```python
from build123d import *
from build123d.topology import SkipClean

# Parameters (mm, degrees)
BOSS_EXTRUDE1_DEPTH = 2
SKETCH3_W           = 30
SKETCH3_H           = 30
SKETCH3_W_2         = 20
SKETCH3_H_2         = 20
BOSS_EXTRUDE2_DEPTH = 10
SKETCH4_W           = 1.5
SKETCH4_H           = 20
BOSS_EXTRUDE3_DEPTH = 1
FILLET2_R           = 1


with BuildPart() as part:
    # Sketch1 → Boss-Extrude1 (new body)
    with BuildSketch(Plane(origin=(0, 0, 0), x_dir=(1, 0, 0), z_dir=(0, 1, 0))):
        Polygon((-12.5, 12.5), (-12.5, -12.5), (-10, -12.5), (-10, 10), (10, 10), (10, -12.5), (12.5, -12.5), (12.5, 12.5), align=None)
    extrude(amount=BOSS_EXTRUDE1_DEPTH)

    # Sketch3 → Boss-Extrude2 (add)
    with BuildSketch(Plane.XZ):
        Rectangle(SKETCH3_W, SKETCH3_H)
        Rectangle(SKETCH3_W_2, SKETCH3_H_2, mode=Mode.SUBTRACT)
    extrude(amount=BOSS_EXTRUDE2_DEPTH)

    # Sketch4 → Boss-Extrude3 (add)
    with BuildSketch(Plane.XZ.offset(10)):
        with Locations((-14.25, 0)):
            Rectangle(SKETCH4_W, SKETCH4_H)
        with Locations((14.25, 0)):
            Rectangle(SKETCH4_W, SKETCH4_H)
    extrude(amount=BOSS_EXTRUDE3_DEPTH)

    # Sketch5 → Cut-Revolve4 (revolve, cut)
    with SkipClean():  # the faces are left unmerged after this step: merging them gives an invalid solid
        with BuildSketch(Plane(origin=(0, 0, 0), x_dir=(0, 0, -1), z_dir=(1, 0, 0))):
            with BuildLine():
                ThreePointArc((-8.75, 0), (-10, 1.25), (-11.25, 0))
                Line((-11.25, 0), (-8.75, 0))
            make_face()
            with BuildLine():
                Line((-8.75, 0), (-11.25, 0))
                ThreePointArc((-11.25, 0), (-10, -1.25), (-8.75, 0))
            make_face()
        revolve(axis=Axis((0, 0, 1000), (0, 0, -1)), mode=Mode.SUBTRACT)
    add(part.part.scale(1), mode=Mode.REPLACE)  # the faces are merged on a copy

    # Fillet2
    fillet2_edges = [part.edges().sort_by_distance(p)[0] for p in [
        (10, -4, -10),
        (-10, -4, -10),
        (-10, 1, 12.5),
        (-12.5, 1, 12.5),
        (-12.5, 1, -12.5),
        (12.5, 1, -12.5),
        (12.5, 1, 12.5),
        (10, 1, 12.5),
        (15, -5, 15),
        (-15, -5, 15),
        (-15, -5, -15),
        (15, -5, -15),
        (-10, -5, 10),
        (10, -5, 10),
    ]]
    fillet(fillet2_edges, radius=FILLET2_R)


solid = part.part
```
For this review, take the finished solid that the model builds, in its own axes (mm). A direction names the side the tool comes from. Round coordinates to 2 decimals unless told otherwise and drop trailing zeros. Order: outer loops, then holes, each group sorted by start corner. A loop starts at its lowest first (then second) coordinate and runs counter-clockwise, first axis right, second up.
Q1. We need section B-B, the plane x = -7.75. Give the boundary of the cut face in (y, z), plus the area to 3 significant figures.
Findings below:
outline: (-10, -15) - (0, -15) - (0, -12.5) - (2, -12.5) - (2, -10) - (-10, -10) - close; (-10, 10) - (0, 10) - (0, 15) - (-10, 15) - close
area: 105 mm2
Q2. Wall thickness on line 1 (Z direction, x = -1.75, y = -9.75); line 2 (X direction, y = 0.75, z = 2): over which ranges is each line inside the solid? List them lowest first.
Findings below:
line 1: z = -15 to -10, 10 to 15
line 2: x = -12.5 to -10, 10 to 12.5
Q3. Machinability: for faces 1 (the flat face through (-14.3, -10.5, -10)), 2 (the flat face through (0, 1, -12.5)), 3 (the cylindrical face through (-12.199, 1.014, -12.215)), 4 (the cylindrical face through (9.699, -4.084, -9.715)), 5 (the flat face through (13.5, -10.5, -0.1)), which of the approach directions +Z, -Z, +X, -X, +Y, -Y give a long, thin tool a straight path to every point of the face, cutting with its end or side? Answer none if there is none.
Findings below:
face 1: -Z, +X, -X, -Y
face 2: -Z, +X, -X, +Y
face 3: -Z, -X, +Y
face 4: +Y, -Y
face 5: +Z, -Z, -Y
Q4. We need section A-A, the plane z = -8.25. Give the boundary of the cut face in (x, y), plus the area to 3 significant figures.
Findings below:
outline: (-15, -11) - (-13.5, -11) - (-13.5, -10) - (-10, -10) - (-10, 2) - (-12.5, 2) - (-12.5, 0) - (-15, 0) - close; (10, -10) - (13.5, -10) - (13.5, -11) - (15, -11) - (15, 0) - (12.5, 0) - (12.5, 2) - (10, 2) - close
area: 113 mm2
Q5. We need section D-D, the plane z = -13. Give the boundary of the cut face in (x, y), plus the area to 3 significant figures.
Findings below:
outline: (-15, -10) - (15, -10) - (15, 0) - (-15, 0) - close
area: 300 mm2
Q6. We need section C-C, the plane y = -7.25. Give the boundary of the cut face in (x, z), plus the area to 3 significant figures.
Findings below:
outline: (-15, -14) arc R1 ccw to (-14, -15) - (14, -15) arc R1 ccw to (15, -14) - (15, 14) arc R1 ccw to (14, 15) - (-14, 15) arc R1 ccw to (-15, 14) - close; hole (-10, -9) arc R1 ccw to (-9, -10) - (9, -10) arc R1 ccw to (10, -9) - (10, 9) arc R1 ccw to (9, 10) - (-9, 10) arc R1 ccw to (-10, 9) - close
area: 500 mm2
Q7. Insertion check: P1, Ø6, axis at x = 10, z = -9, coming from the -Y side; P2, Ø0.6, axis at y = 1, z = -5.5, coming from the -X side. Each pin has a flat end and moves straight along its axis. Give the tip position at first contact, or say it passes through.
Findings below:
P1: stops at y = -10
P2: stops at x = -12.5
Q8. Mouldability with a two-part tool opening along Z and no side actions: class faces 6 (the cylindrical face through (-12.215, 1.014, 12.199)), 7 (the flat face through (10, -4, 1)), 8 (the flat face through (-12.5, 1, 0)) as pulls with the +Z half, pulls with the -Z half, needs draft (parallel to the pull), parting line crosses it, or undercut.
Findings below:
face 6: pulls with the +Z half
face 7: undercut
face 8: needs draft
